The listing builds one solid part. Answer for the finished solid, in the listing's coordinates (mm). A direction names the side the tool comes from. Give positions to 0.01 mm unless a question says otherwise; leave off trailing zeros. Loops run counter-clockwise (first coordinate to the right, second up) from the corner with the lowest first, then second, coordinate; pieces in that order, holes last. Notation, with made-up numbers: (63.25, 55.25) - (115.25, 55.25) arc R24 ccw to (115.25, 86.25) - close; hole circle Ø3 at (-38.5, 13). An arc over 180 degrees is marked (long way). One line per item, written item: value. Start each with the question number.
from build123d import *

# Parameters (mm, degrees)
SKETCH1_R           = 12.7
EXTRUDE1_DEPTH      = 159.512
SKETCH3_R           = 10.8204
CUT_EXTRUDE1_DEPTH  = 114.808
SKETCH4_R           = 9.017
CUT_EXTRUDE2_DEPTH  = 45.704
CHAMFER1_SIZE       = 1.778
CHAMFER2_SIZE       = 0.762
CHAMFER2_SIZE2      = 0.508
SKETCH5_R           = 9.5758
CUT_EXTRUDE3_DEPTH  = 29.21
SKETCH8_R           = 10.287
CUT_EXTRUDE5_DEPTH  = 25.273
SKETCH9_R           = 11.0871
CUT_EXTRUDE6_DEPTH  = 18.1864
CHAMFER3_SIZE       = 10.3632
CHAMFER3_SIZE2      = 0.7239
CUT_EXTRUDE7_DEPTH  = 7.62
SKETCH11_R          = 2.032
CUT_EXTRUDE11_DEPTH = 3.302
SKETCH15_R          = 1.7018
CUT_EXTRUDE12_DEPTH = 3.302
SKETCH16_R          = 9.525
CUT_EXTRUDE13_DEPTH = 12.7
SKETCH17_R          = 2.032
CUT_EXTRUDE14_DEPTH = 3.302
SKETCH18_R          = 1.7018
CUT_EXTRUDE15_DEPTH = 3.302


with BuildPart() as part:
    # Sketch1 → Extrude1 (new body)
    with BuildSketch(Plane.XY):
        Circle(SKETCH1_R)
    extrude(amount=EXTRUDE1_DEPTH)

    # Sketch3 → Cut-Extrude1 (cut)
    with BuildSketch(Plane(origin=(0, 0, 0), x_dir=(-1, 0, 0), z_dir=(0, 0, -1))):
        Circle(SKETCH3_R)
    extrude(amount=-CUT_EXTRUDE1_DEPTH, mode=Mode.SUBTRACT)

    # Sketch4 → Cut-Extrude2 (cut, through all)
    with BuildSketch(Plane(origin=(0, 0, 114.808), x_dir=(-1, 0, 0), z_dir=(0, 0, -1))):
        Circle(SKETCH4_R)
    extrude(amount=-CUT_EXTRUDE2_DEPTH, mode=Mode.SUBTRACT)

    # Chamfer1
    chamfer1_edges = [part.edges().sort_by_distance(p)[0] for p in [
        (9.017, 0, 114.808),
    ]]
    chamfer(chamfer1_edges, length=CHAMFER1_SIZE)

    # Chamfer2
    chamfer2_edges = [part.edges().sort_by_distance(p)[0] for p in [
        (9.017, 0, 116.586),
    ]]
    chamfer2_side = [part.faces().sort_by_distance(p)[0] for p in [
        (9.906, 0, 115.697),
    ]]
    chamfer(chamfer2_edges, length=CHAMFER2_SIZE, length2=CHAMFER2_SIZE2, reference=chamfer2_side[0])

    # Sketch5 → Cut-Extrude3 (cut)
    with BuildSketch(Plane.XY.offset(159.512)):
        Circle(SKETCH5_R)
    extrude(amount=-CUT_EXTRUDE3_DEPTH, mode=Mode.SUBTRACT)

    # Sketch8 → Cut-Extrude5 (cut)
    with BuildSketch(Plane.XY.offset(159.512)):
        Circle(SKETCH8_R)
    extrude(amount=-CUT_EXTRUDE5_DEPTH, mode=Mode.SUBTRACT)

    # Sketch9 → Cut-Extrude6 (cut)
    with BuildSketch(Plane.XY.offset(159.512)):
        Circle(SKETCH9_R)
    extrude(amount=-CUT_EXTRUDE6_DEPTH, mode=Mode.SUBTRACT)

    # Chamfer3
    chamfer3_edges = [part.edges().sort_by_distance(p)[0] for p in [
        (-12.7, 0, 159.512),
    ]]
    chamfer3_side = [part.faces().sort_by_distance(p)[0] for p in [
        (-12.7, 0, 79.756),
    ]]
    chamfer(chamfer3_edges, length=CHAMFER3_SIZE, length2=CHAMFER3_SIZE2, reference=chamfer3_side[0])

    # Sketch10 → Cut-Extrude7 (cut)
    with BuildSketch(Plane(origin=(0, -12.7, 0), x_dir=(-1, 0, 0), z_dir=(0, 1, 0))):
        with BuildLine():
            Line((2.3114, 0), (2.3114, 72.0725))
            ThreePointArc((2.3114, 72.0725), (2.776367985, 73.195032015), (3.8989, 73.66))
            Line((3.8989, 73.66), (5.4991, 73.66))
            ThreePointArc((5.4991, 73.66), (6.621632015, 74.124967985), (7.0866, 75.2475))
            Line((7.0866, 75.2475), (7.0866, 107.6325))
            ThreePointArc((7.0866, 107.6325), (6.621632015, 108.755032015), (5.4991, 109.22))
            Line((5.4991, 109.22), (3.3401, 109.22))
            ThreePointArc((3.3401, 109.22), (2.217567985, 108.755032015), (1.7526, 107.6325))
            Line((1.7526, 107.6325), (1.7526, 98.1075))
            ThreePointArc((1.7526, 98.1075), (1.287632015, 96.984967985), (0.1651, 96.52))
            Line((0.1651, 96.52), (-0.7239, 96.52))
            ThreePointArc((-0.7239, 96.52), (-1.846432015, 96.055032015), (-2.3114, 94.9325))
            Line((-2.3114, 94.9325), (-2.3114, 0))
            Line((-2.3114, 0), (2.3114, 0))
        make_face()
    extrude(amount=CUT_EXTRUDE7_DEPTH, mode=Mode.SUBTRACT)

    # Sketch11 → Cut-Extrude11 (cut)
    with BuildSketch(Plane(origin=(0, -12.7, 0), x_dir=(-1, 0, 0), z_dir=(0, 1, 0))):
        with Locations(Location((0, 126.619, 0), (0, 0, 270))):  # turned: the seam where the file's is
            Circle(SKETCH11_R)
    extrude(amount=CUT_EXTRUDE11_DEPTH, mode=Mode.SUBTRACT)

    # Sketch15 → Cut-Extrude12 (cut)
    with BuildSketch(Plane.XZ.offset(9.398)):
        with Locations(Location((0, 126.619, 0), (0, 0, 270))):  # turned: the seam where the file's is
            Circle(SKETCH15_R)
    extrude(amount=-CUT_EXTRUDE12_DEPTH, mode=Mode.SUBTRACT)

    # Sketch16 → Cut-Extrude13 (cut)
    with BuildSketch(Plane(origin=(0, 12.7, 0), x_dir=(-1, 0, 0), z_dir=(0, 1, 0))):
        with Locations(Location((0, 105.9688, 0), (0, 0, 90))):  # turned: the seam where the file's is
            Circle(SKETCH16_R)
    extrude(amount=-CUT_EXTRUDE13_DEPTH, mode=Mode.SUBTRACT)

    # Sketch17 → Cut-Extrude14 (cut)
    with BuildSketch(Plane(origin=(0, 12.7, 0), x_dir=(-1, 0, 0), z_dir=(0, 1, 0))):
        with Locations(Location((0, 122.682, 0), (0, 0, 90))):  # turned: the seam where the file's is
            Circle(SKETCH17_R)
    extrude(amount=-CUT_EXTRUDE14_DEPTH, mode=Mode.SUBTRACT)

    # Sketch18 → Cut-Extrude15 (cut)
    with BuildSketch(Plane(origin=(0, 9.398, 0), x_dir=(-1, 0, 0), z_dir=(0, 1, 0))):
        with Locations(Location((0, 122.682, 0), (0, 0, 90))):  # turned: the seam where the file's is
            Circle(SKETCH18_R)
    extrude(amount=-CUT_EXTRUDE15_DEPTH, mode=Mode.SUBTRACT)


solid = part.part
1. A cutting plane is placed at B-B (x = 6). Give the number of separate pieces and of enclosed holes in the cut face, plus the area to 3 significant figures.
2. For faces 1 (the cylindrical face through (1.43, -9.19, 125.7)), 2 (the cylindrical face through (-1.984, 11.072, 122.242)), 3 (the cylindrical face through (10.81, 0.48, 56.6)), 4 (the cylindrical face through (-8.798, -6.746, 150.546)), determine the directions among +Z, -Z, +X, -X, +Y, -Y from which every point of the face is accessible in a straight line to the end or side of a thin tool.
3. A cutting plane is placed at A-A (z = 79). Determine the outline of the cut face in (x, y).
4. Find the intervals of material crossed by L1, parallel to X at y = -3, z = 119; L2, parallel to Y at x = 0, z = 82; L3, parallel to Y at x = 0, z = 154, in increasing order. Write a range as [from, to].
5. Determine the mould class of faces 5 (the flat face through (3, -11, 159.512)), 6 (the conical face through (11.687, 3.68, 155.554)), 7 (the flat face through (7, -7, 134.239)) for opening direction X: released by +X, released by -X, zero draft, split by the parting line, or undercut.
6. Flat-ended cylindrical pins translate along their axes: pin 1 (0.7 mm diameter, centred on y = -9, z = 86.5, fed in from +X); pin 2 (1.5 mm diameter, centred on y = -11.5, z = 103, fed in from -X); pin 3 (1 mm diameter, centred on y = -11.5, z = 55, fed in from -X); pin 4 (11 mm diameter, centred on x = 0, y = 0, fed in from +Z). Find the tip coordinate at first contact, or state that the pin passes through.
7. A cutting plane is placed at C-C (z = 50.5). Determine the outline of the cut face in (x, y).
Results below:
1. separate pieces: 3
1. enclosed holes: 0
1. area: 733 mm^2
2. face 1: -Y
2. face 2: +Y
2. face 3: -Z
2. face 4: +Z
3. outline: (-7.09, -10.54) - (-7.09, -8.18) arc R10.82 cw (long way) to (2.31, -10.57) - (2.31, -12.49) arc R12.7 ccw (long way) to start
4. L1: x = [-12.34, -8.5], [8.5, 12.34]
4. L2: y = [10.82, 12.7]
4. L3: y = [-12.36, -11.09], [11.09, 12.36]
5. face 5: zero draft
5. face 6: split by the parting line
5. face 7: undercut
6. pin 1: stops at x = 9.3
6. pin 2: stops at x = -1.75
6. pin 3: stops at x = -6.35
6. pin 4: passes through
7. outline: (-2.31, -12.49) - (-2.31, -10.57) arc R10.82 cw (long way) to (2.31, -10.57) - (2.31, -12.49) arc R12.7 ccw (long way) to start
